Work out the finished part from the listing and answer in its coordinate system (mm). A direction names the side the tool comes from. Coordinates: 2 decimals unless noted, no trailing zeros. Loops run counter-clockwise (first coordinate to the right, second up) from the corner with the lowest first, then second, coordinate; pieces in that order, holes last. Notation, with made-up numbers: (-31.75, -12.75) - (-25.75, -12.75) arc R16 ccw to (-25.75, 17.25) - close; hole circle Ø3 at (-8.75, 12.25). An arc over 180 degrees is marked (long way). Write each question's results on one line, items separated by ' | '. Start each with the question number.
1. A cutting plane is placed at A-A on x = 37. Determine the outline of the cut face in (y, z).
2. Each of these flat-tipped pins is pushed along its axis until it touches: P1, Ø2.5, axis at x = 34.06, y = -35.75, coming from the +Z side; P2, Ø10, axis at y = -13.5, z = 8, coming from the -X side; P3, Ø3.5, axis at x = 35.5, z = 10.5, coming from the -Y side. Where does it stop, or does it pass through?
3. A cutting plane is placed at C-C on z = 12.5. Determine the outline of the cut face in (x, y), then the cut area to 3 significant figures.
4. A cutting plane is placed at D-D on x = 9. Determine the outline of the cut face in (y, z), then the cut area to 3 significant figures.
5. Determine the mould class of faces 1 (the flat face through (35, -8, 16.002)), 2 (the flat face through (17, 0, 12.4)), 3 (the flat face through (28.062, -21, 10)) for opening direction Y: released by +Y, released by -Y, zero draft, split by the parting line, or undercut.
6. Find the intervals of material crossed by line 1 along Y through (x, z) = (31, 14.25); line 2 along Y through (x, z) = (15, 4.25); line 3 along X through (y, z) = (-2.6, 10) (3 decimals), in increasing order. Write a range as [from, to].
7. Which of the six approach directions +Z, -Z, +X, -X, +Y, -Y give full straight-line access (tool end or side, diameter ignored) to faces 4 (the flat face through (35, -39, 10)), 5 (the flat face through (35, -8, 3.998)), 6 (the flat face through (12, -39, 10)), 7 (the cylindrical face through (33.063, -7.206, 11.072))?
from build123d import *

# Parameters (mm, degrees)
EXTRUDE_1_DEPTH     = 20
CUT_EXTRUDE_2_DEPTH = 20
SKETCH_6_W          = 20
SKETCH_6_H          = 46
EXTRUDE_2_DEPTH     = 3
SKETCH_7_W          = 4
SKETCH_7_H          = 38
CUT_EXTRUDE_4_DEPTH = 23
SKETCH_8_W          = 27.047351985
SKETCH_8_H          = 20
EXTRUDE_3_DEPTH     = 3
SKETCH_9_W          = 28.062086438
SKETCH_9_H          = 3
CUT_EXTRUDE_5_DEPTH = 50
CUT_EXTRUDE_6_DEPTH = 50
SKETCH_11_W         = 6.001651559
SKETCH_11_H         = 4
EXTRUDE_4_DEPTH     = 15
SKETCH_16_W         = 14.934651965
SKETCH_16_H         = 12.003303118
EXTRUDE_5_DEPTH     = 2
SKETCH_21_R         = 1
CUT_EXTRUDE_8_DEPTH = 10


with BuildPart() as part:
    # 草图1 → 凸台-拉伸1 (new body)
    with BuildSketch(Plane.XY):
        Polygon((25.062086438, -46), (25.062086438, 0), (0, 0), (0, -4), (20, -4), (20, -42), (0, -42), (0, -46), align=None)
    extrude(amount=EXTRUDE_1_DEPTH)

    # 草图3 → 切除-拉伸2 (cut)
    with BuildSketch(Plane(origin=(0, 0, 0), x_dir=(1, 0, 0), z_dir=(0, 1, 0))):
        with BuildLine():
            Line((5.429347826, -13.448374319), (21.170329997, -11.4885069))
            ThreePointArc((21.170329997, -11.4885069), (22.485, -10), (21.170329997, -8.5114931))
            Line((21.170329997, -8.5114931), (5.429347826, -6.551625681))
            ThreePointArc((5.429347826, -6.551625681), (1.525, -10), (5.429347826, -13.448374319))
        make_face()
    extrude(amount=-CUT_EXTRUDE_2_DEPTH, mode=Mode.SUBTRACT)

    # 草图6 → 凸台-拉伸2 (add)
    with BuildSketch(Plane(origin=(25.062086438, 0, 0), x_dir=(0, 0, -1), z_dir=(1, 0, 0))):
        with Locations((-10, -23)):
            Rectangle(SKETCH_6_W, SKETCH_6_H)
    extrude(amount=EXTRUDE_2_DEPTH)

    # 草图7 → 切除-拉伸4 (cut)
    with BuildSketch(Plane.XY.offset(20)):
        with Locations((22, -23)):
            Rectangle(SKETCH_7_W, SKETCH_7_H)
    extrude(amount=-CUT_EXTRUDE_4_DEPTH, mode=Mode.SUBTRACT)

    # 草图8 → 凸台-拉伸3 (add)
    with BuildSketch(Plane(origin=(0, -42, 0), x_dir=(1, 0, 0), z_dir=(0, 1, 0))):
        with Locations((13.523675993, -10)):
            Rectangle(SKETCH_8_W, SKETCH_8_H)
    extrude(amount=EXTRUDE_3_DEPTH)

    # 草图9 → 切除-拉伸5 (cut)
    with BuildSketch(Plane.XY.offset(20)):
        with Locations((14.031043219, -44.5)):
            Rectangle(SKETCH_9_W, SKETCH_9_H)
    extrude(amount=-CUT_EXTRUDE_5_DEPTH, mode=Mode.SUBTRACT)

    # 草图10 → 切除-拉伸6 (cut)
    with BuildSketch(Plane(origin=(0, 0, 0), x_dir=(1, 0, 0), z_dir=(0, 1, 0))):
        with BuildLine():
            Line((10, 0), (0, 0))
            Line((0, 0), (0, -10))
            ThreePointArc((0, -10), (2.928932188, -2.928932188), (10, 0))
        make_face()
        with BuildLine():
            ThreePointArc((10, -20), (2.928932188, -17.071067812), (0, -10))
            Line((0, -10), (0, -20))
            Line((0, -20), (10, -20))
        make_face()
    extrude(amount=-CUT_EXTRUDE_6_DEPTH, mode=Mode.SUBTRACT)

    # 草图11 → 凸台-拉伸4 (add)
    with BuildSketch(Plane(origin=(28.062086438, 0, 0), x_dir=(0, 0, -1), z_dir=(1, 0, 0))):
        with Locations((-13.00082578, -8)):
            Rectangle(SKETCH_11_W, SKETCH_11_H)
        with Locations((-6.999174221, -8)):
            Rectangle(SKETCH_11_W, SKETCH_11_H)
        with Locations((-6.999174221, -35)):
            Rectangle(SKETCH_11_W, SKETCH_11_H)
        with Locations((-13.00082578, -35)):
            Rectangle(SKETCH_11_W, SKETCH_11_H)
    extrude(amount=EXTRUDE_4_DEPTH)

    # 草图16 → 凸台-拉伸5 (add)
    with BuildSketch(Plane.XZ.offset(37)):
        with Locations((35.529412421, 10)):
            Rectangle(SKETCH_16_W, SKETCH_16_H)
    extrude(amount=EXTRUDE_5_DEPTH)

    # 草图21 → 切除-拉伸8 (cut)
    with BuildSketch(Plane.XY.offset(16.001651559)):
        with Locations((34.062086438, -7.25)):
            Circle(SKETCH_21_R)
        with Locations((34.062086438, -35.75)):
            Circle(SKETCH_21_R)
    extrude(amount=-CUT_EXTRUDE_8_DEPTH, mode=Mode.SUBTRACT)


solid = part.part
Values:
1) outline: (-39, 4) - (-33, 4) - (-33, 16) - (-39, 16) - close; (-10, 4) - (-6, 4) - (-6, 16) - (-10, 16) - close
2) P1: z = 16 | P2: x = 24 | P3: y = -39
3) outline: (0.32, -43) - (28.06, -43) - (28.06, -39) - (43, -39) - (43, -37) - (43.06, -37) - (43.06, -33) - (28.06, -33) - (28.06, -10) - (43.06, -10) - (43.06, -6) - (28.06, -6) - (28.06, 0) - (13.05, 0) - (13.05, -4) - (24, -4) - (24, -39) - (0.32, -39) - close; (0.32, -4) - (2.59, -4) - (2.59, 0) - (0.32, 0) - close; hole circle Ø2 at (34.06, -35.75); hole circle Ø2 at (34.06, -7.25) | area: 466 mm^2
4) outline: (-43, 0.05) - (-39, 0.05) - (-39, 19.95) - (-43, 19.95) - close; (-4, 0.05) - (0, 0.05) - (0, 7) - (-4, 7) - close; (-4, 13) - (0, 13) - (0, 19.95) - (-4, 19.95) - close | area: 135 mm^2
5) face 1: zero draft | face 2: released by +Y | face 3: undercut
6) line 1: [-39, -33], [-10, -6] | line 2: [-43, -39], [-4, 0] | line 3: [0, 1.525], [22.485, 28.062]
7) face 4: +Z, -Z, +X, -Y | face 5: -Z, +X, +Y, -Y | face 6: +Z, -Z, -X | face 7: +Z
